Could you check a few things on this drawing? It's one solid part, dimensions in mm from its lowest x, y, z. A direction names the side the tool comes from. Coordinates: 2 decimals unless noted, no trailing zeros. Order: outer loops, then holes, each group sorted by start corner. A loop starts at its lowest first (then second) coordinate and runs counter-clockwise, first axis right, second up.
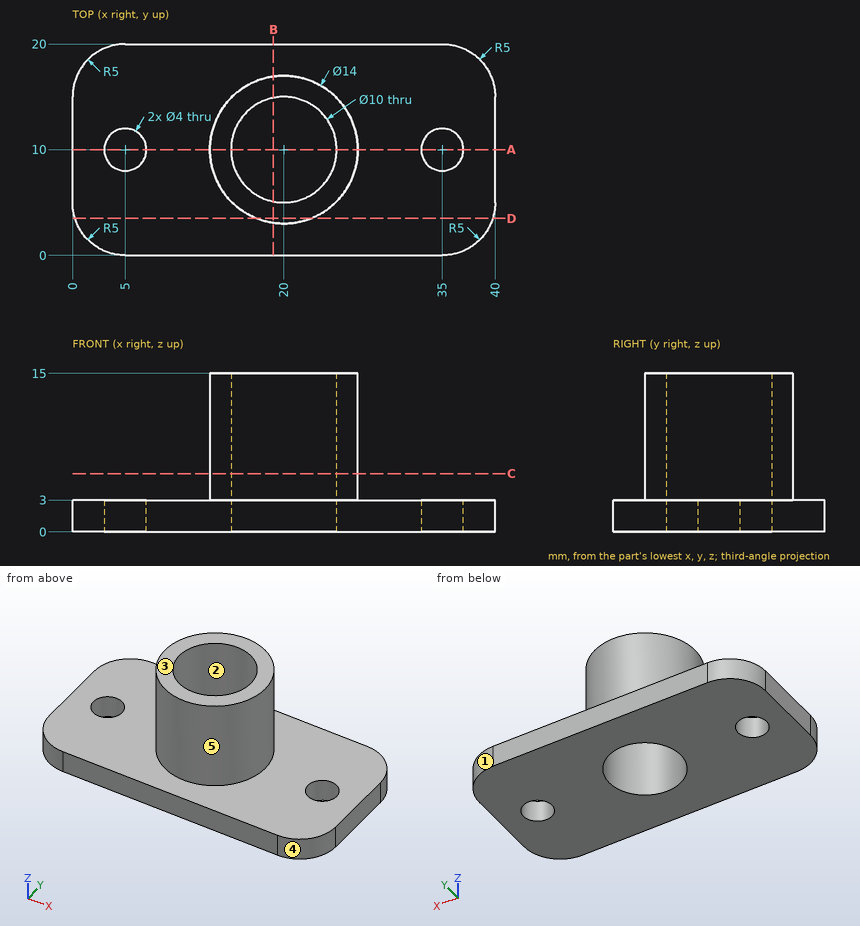
Q1. For the marked faces 4 and 5, which set-ups out of +Z, -Z, +X, -X, +Y, -Y let a thin tool reach every point of the face, with its end or its side?
Q2. If we section it at D-D on y = 3.5: Write out the boundary of the cut face in (x, z), then the cut area to 3 significant figures.
Q3. If we section it at B-B on x = 19: Write out the boundary of the cut face in (y, z), then the cut area to 3 significant figures.
Q4. If we section it at C-C on z = 5.5: Write out the boundary of the cut face in (x, y), then the cut area to 3 significant figures.
Q5. If we section it at A-A on y = 10: Write out the boundary of the cut face in (x, z).
Q6. Will these pins go through, and if not, where does the flat tip stop? pin 1 (6 mm diameter, centred on x = 12.5, z = 10.5, fed in from +Y); pin 2 (1 mm diameter, centred on y = 3.5, z = 8, fed in from +X); pin 3 (4 mm diameter, centred on y = 10, z = 13.5, fed in from +X).
Q7. We'd pull the mould along Y, two halves only. Please class the marked faces 1, 2 and 3: pulls with the +Y half, pulls with the -Y half, needs draft (parallel to the pull), parting line crosses it, or undercut.
Q8. I need wall thicknesses on L1, parallel to X at y = 10.75, z = 1.75; L2, parallel to Y at x = 35, z = 1.25; L3, parallel to Z at x = 13.5, y = 14. Which ranges of each line are inside material? Lowest first, please.
Reply:
1. face 4: +Z, -Z, +X, -Y
1. face 5: +Z
2. outline: (0.23, 0) - (39.77, 0) - (39.77, 3) - (22.6, 3) - (22.6, 15) - (17.4, 15) - (17.4, 3) - (0.23, 3) - close
2. area: 181 mm2
3. outline: (0, 0) - (5.1, 0) - (5.1, 15) - (3.07, 15) - (3.07, 3) - (0, 3) - close; (14.9, 0) - (20, 0) - (20, 3) - (16.93, 3) - (16.93, 15) - (14.9, 15) - close
3. area: 79.3 mm2
4. outline: circle Ø14 at (20, 10); hole circle Ø10 at (20, 10)
4. area: 75.4 mm2
5. outline: (0, 0) - (3, 0) - (3, 3) - (0, 3) - close; (7, 0) - (15, 0) - (15, 15) - (13, 15) - (13, 3) - (7, 3) - close; (25, 0) - (33, 0) - (33, 3) - (27, 3) - (27, 15) - (25, 15) - close; (37, 0) - (40, 0) - (40, 3) - (37, 3) - close
6. pin 1: stops at y = 15.36
6. pin 2: stops at x = 23.61
6. pin 3: stops at x = 27
7. face 1: pulls with the +Y half
7. face 2: undercut
7. face 3: needs draft
8. L1: x = 0 to 3.15, 6.85 to 15.06, 24.94 to 33.15, 36.85 to 40
8. L2: y = 0 to 8, 12 to 20
8. L3: z = 0 to 3
